Geometry: see drawing. Coordinates: mm, zero at the bounding-box minimum. A direction names the side the tool comes from. Give positions to 0.01 mm unless a question says otherwise; leave off trailing zeros. Write each loop counter-clockwise with the first axis right and the second up, starting at its lowest first coordinate (ties: lowest second). Pieces come first, ordered by that corner, then holes. Notation, with made-up numbers: (59, -26) -> (104, -26) arc R13 ccw to (104, -15) -> close; hole circle Ø5 at (61.25, 51.25). An arc over 180 degrees is marked (long way). Write item = value, one per line.
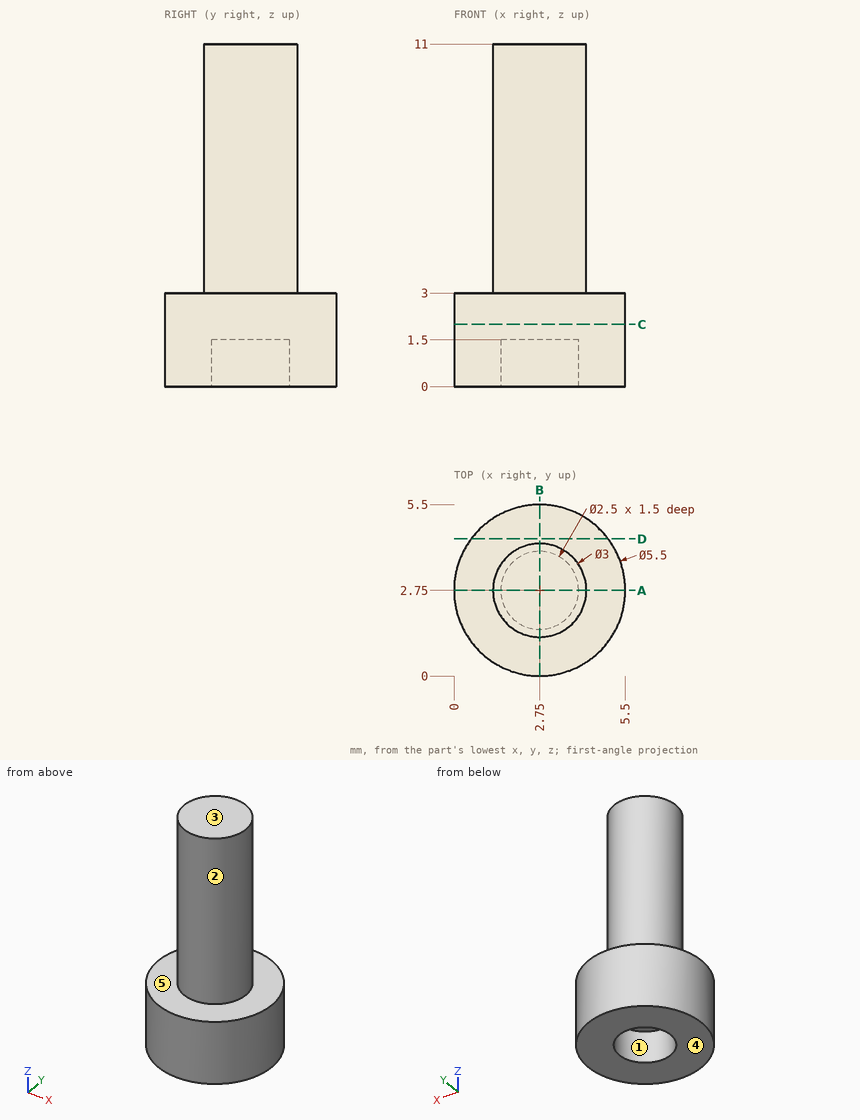
(1) Material intervals for line 1 (Y direction, x = 2.75, z = 0.4); line 2 (Z direction, x = 4.25, y = 4); line 3 (Z direction, x = 3.6, y = 3), sorted ascending.
Values follow:
line_1 = 0 to 1.5, 4 to 5.5
line_2 = 0 to 3
line_3 = 1.5 to 11
(2) Section query A-A (y = 2.75). Return loops of the section in (x, z), plus the area to 4 significant figures.
Values follow:
outline = (0, 0) -> (1.5, 0) -> (1.5, 1.5) -> (4, 1.5) -> (4, 0) -> (5.5, 0) -> (5.5, 3) -> (4.25, 3) -> (4.25, 11) -> (1.25, 11) -> (1.25, 3) -> (0, 3) -> close
area = 36.75 mm2
(3) Section query C-C (z = 2). Return loops of the section in (x, y).
Values follow:
outline = circle Ø5.5 at (2.75, 2.75)
(4) Access query for the marked faces 4 and 5. Directions: +Z, -Z, +X, -X, +Y, -Y. A direction counts if a zero-diameter tool reaches every point of the face in a straight line with its end or side. Return the directions, or none.
Values follow:
face_4 = -Z, +X, -X, +Y, -Y
face_5 = +Z
(5) Section query D-D (y = 4.4). Return loops of the section in (x, z), plus the area to 3 significant figures.
Values follow:
outline = (0.55, 0) -> (4.95, 0) -> (4.95, 3) -> (0.55, 3) -> close
area = 13.2 mm2
(6) Pull-direction query (X, two-part tool) for the marked faces 1, 2 and 3; classes: pulls with the +X half, pulls with the -X half, needs draft (parallel to the pull), parting line crosses it, or undercut.
Values follow:
face_1 = undercut
face_2 = parting line crosses it
face_3 = needs draft
(7) First-contact query: pin 1 (2 mm diameter, centred on x = 2.75, y = 2.75, fed in from -Z); pin 2 (1 mm diameter, centred on x = 1.5, z = 3, fed in from +Y); pin 3 (1.5 mm diameter, centred on y = 2.5, z = 4, fed in from +X). Flat tips, straight axial feed; report the tip coordinate or a pass-through.
Values follow:
pin_1 = 1.5
pin_2 = 5.4
pin_3 = 4.25
